Could you check a few things on this drawing? It's one solid part, dimensions in mm from its lowest x, y, z. Give positions to 0.01 mm unless a question says otherwise; leave off trailing zeros. Order: outer loops, then holes, each group sorted by start corner. A loop starts at its lowest first (then second) coordinate and runs counter-clockwise, first axis right, second up.
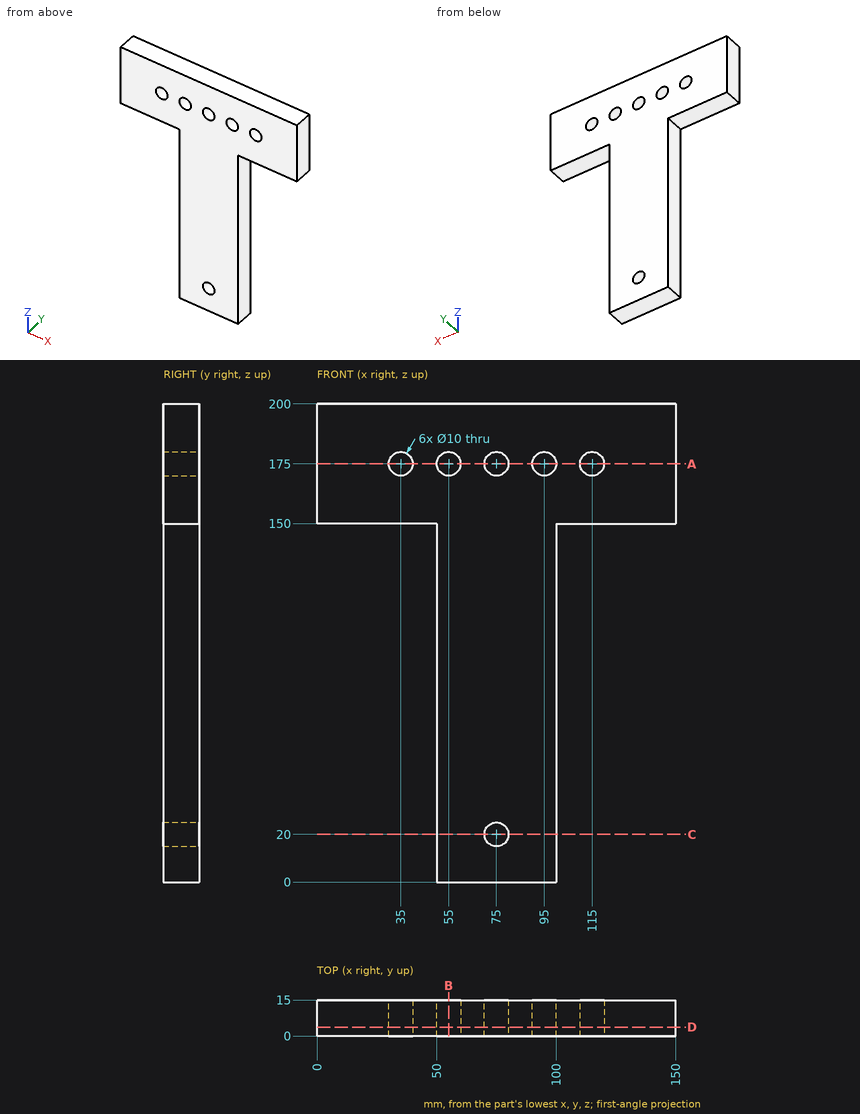
Q1. I'm going to push flat-ended pins straight in: P1, Ø3, axis at y = 3.5, z = 103.5, coming from the +X side; P2, Ø4.5, axis at y = 10.5, z = 40.5, coming from the -X side. Where does each tip first touch, or does it pass through?
Filled sheet:
P1: stops at x = 100
P2: stops at x = 50
Q2. If we section it at A-A on z = 175: List the corners of the cut face in (x, y) for me.
Filled sheet:
outline: (0, 0) - (30, 0) - (30, 15) - (0, 15) - close; (40, 0) - (50, 0) - (50, 15) - (40, 15) - close; (60, 0) - (70, 0) - (70, 15) - (60, 15) - close; (80, 0) - (90, 0) - (90, 15) - (80, 15) - close; (100, 0) - (110, 0) - (110, 15) - (100, 15) - close; (120, 0) - (150, 0) - (150, 15) - (120, 15) - close
Q3. If we section it at D-D on y = 3.75: List the corners of the cut face in (x, z) for me.
Filled sheet:
outline: (0, 150) - (50, 150) - (50, 0) - (100, 0) - (100, 150) - (150, 150) - (150, 200) - (0, 200) - close; hole circle Ø10 at (35, 175); hole circle Ø10 at (55, 175); hole circle Ø10 at (75, 20); hole circle Ø10 at (75, 175); hole circle Ø10 at (95, 175); hole circle Ø10 at (115, 175)
Q4. If we section it at B-B on x = 55: List the corners of the cut face in (y, z) for me, plus the area to 3 significant figures.
Filled sheet:
outline: (0, 0) - (15, 0) - (15, 170) - (0, 170) - close; (0, 180) - (15, 180) - (15, 200) - (0, 200) - close
area: 2,850 mm2
Q5. I need wall thicknesses on L1, parallel to X at y = 7.25, z = 175; L2, parallel to Z at x = 75, y = 8; L3, parallel to Z at x = 35, y = 11.25. Which ranges of each line are inside material? Lowest first, please.
Filled sheet:
L1: x = 0 to 30, 40 to 50, 60 to 70, 80 to 90, 100 to 110, 120 to 150
L2: z = 0 to 15, 25 to 170, 180 to 200
L3: z = 150 to 170, 180 to 200
Q6. If we section it at C-C on z = 20: List the corners of the cut face in (x, y) for me, plus the area to 3 significant figures.
Filled sheet:
outline: (50, 0) - (70, 0) - (70, 15) - (50, 15) - close; (80, 0) - (100, 0) - (100, 15) - (80, 15) - close
area: 600 mm2
